Could you check a few things on this model? Use its own coordinates, in mm. Face numbers are marked on the shaded views. A direction names the side the tool comes from. Round coordinates to 2 decimals unless told otherwise and drop trailing zeros. Write each loop counter-clockwise with the first axis right and the second up, starting at its lowest first coordinate (ties: lowest second). Pieces come first, ordered by that corner, then holes. Notation, with made-up numbers: (-2.5, -23.5) -> (3.5, -23.5) arc R20 ccw to (3.5, 7.5) -> close; hole circle Ø4 at (39, 33). An arc over 180 degrees is marked (long way). Answer in a Markdown table with one row per item.
from build123d import *

# Parameters (mm, degrees)
BOSS_EXTRUDE7_DEPTH     = 6.5
BOSS_EXTRUDE8_START     = 1.7
BOSS_EXTRUDE8_DEPTH     = 1.7
CUT_EXTRUDE1_DEPTH      = 8.5
SKETCH6_W               = 12
SKETCH6_H               = 7.5
CUT_EXTRUDE2_DEPTH      = 8.5
CHAMFER1_SIZE           = 0.8
CHAMFER1_SIZE2          = 1.231891971
SKETCH7_R               = 0.4
CUT_EXTRUDE3_DEPTH      = 2
CUT_EXTRUDE3_DEPTH_BACK = 36.03740858
CHAMFER2_SIZE           = 0.5
CUT_EXTRUDE4_REACH      = 34.411
SKETCH12_R              = 0.8
BOSS_EXTRUDE9_DEPTH     = 0.5
CHAMFER3_SIZE           = 0.5


# Some blends are built 0.0001 mm under size
with BuildPart() as part:
    # Sketch1 → Boss-Extrude7 (new body)
    with BuildSketch(Plane(origin=(0, 0, 0), x_dir=(1, 0, 0), z_dir=(0, 1, 0))):
        with BuildLine():
            Line((0.8, 26.4), (19.9, 26.4))
            ThreePointArc((19.9, 26.4), (21.455634919, 25.755634919), (22.1, 24.2))
            Line((22.1, 24.2), (22.1, 0.8))
            ThreePointArc((22.1, 0.8), (21.455634919, -0.755634919), (19.9, -1.4))
            Line((19.9, -1.4), (0.8, -1.4))
            ThreePointArc((0.8, -1.4), (-0.755634919, -0.755634919), (-1.4, 0.8))
            Line((-1.4, 0.8), (-1.4, 24.2))
            ThreePointArc((-1.4, 24.2), (-0.755634919, 25.755634919), (0.8, 26.4))
        make_face()
        with BuildLine():
            Line((0.8, 25.2), (19.9, 25.2))
            ThreePointArc((19.9, 25.2), (20.607106781, 24.907106781), (20.9, 24.2))
            Line((20.9, 24.2), (20.9, 0.8))
            ThreePointArc((20.9, 0.8), (20.607106781, 0.092893219), (19.9, -0.2))
            Line((19.9, -0.2), (0.8, -0.2))
            ThreePointArc((0.8, -0.2), (0.092893219, 0.092893219), (-0.2, 0.8))
            Line((-0.2, 0.8), (-0.2, 24.2))
            ThreePointArc((-0.2, 24.2), (0.092893219, 24.907106781), (0.8, 25.2))
        make_face(mode=Mode.SUBTRACT)
    extrude(amount=BOSS_EXTRUDE7_DEPTH)

    # Sketch4 → Boss-Extrude8 (add)
    with BuildSketch(Plane.XZ.offset(BOSS_EXTRUDE8_START)):
        with BuildLine():
            Line((0.8, -26.4), (19.9, -26.4))
            ThreePointArc((19.9, -26.4), (21.455634919, -25.755634919), (22.1, -24.2))
            Line((22.1, -24.2), (22.1, -0.8))
            ThreePointArc((22.1, -0.8), (21.455634919, 0.755634919), (19.9, 1.4))
            Line((19.9, 1.4), (0.8, 1.4))
            ThreePointArc((0.8, 1.4), (-0.755634919, 0.755634919), (-1.4, -0.8))
            Line((-1.4, -0.8), (-1.4, -24.2))
            ThreePointArc((-1.4, -24.2), (-0.755634919, -25.755634919), (0.8, -26.4))
        make_face()
    extrude(amount=-BOSS_EXTRUDE8_DEPTH)

    # Sketch5 → Cut-Extrude1 (cut)
    with BuildSketch(Plane(origin=(0, 0, -26.4), x_dir=(-1, 0, 0), z_dir=(0, 0, -1))):
        with BuildLine():
            Line((-13.25, 2.9), (-7.45, 2.9))
            ThreePointArc((-7.45, 2.9), (-5.75, 1.2), (-7.45, -0.5))
            Line((-7.45, -0.5), (-13.25, -0.5))
            ThreePointArc((-13.25, -0.5), (-14.95, 1.2), (-13.25, 2.9))
        make_face()
    extrude(amount=-CUT_EXTRUDE1_DEPTH, mode=Mode.SUBTRACT)

    # Sketch6 → Cut-Extrude2 (cut)
    with BuildSketch(Plane(origin=(0, 0, 0), x_dir=(1, 0, 0), z_dir=(0, 1, 0))):
        with Locations((10.35, 9.85)):
            Rectangle(SKETCH6_W, SKETCH6_H)
    extrude(amount=-CUT_EXTRUDE2_DEPTH, mode=Mode.SUBTRACT)

    # Chamfer1
    chamfer1_edges = [part.edges().sort_by_distance(p)[0] for p in [
        (10.35, -1.7, -6.1),
        (16.35, -1.7, -9.85),
        (10.35, -1.7, -13.6),
        (4.35, -1.7, -9.85),
    ]]
    chamfer1_side = [part.faces().sort_by_distance(p)[0] for p in [
        (-0.498235424, -1.7, -25.498235424),
    ]]
    chamfer(chamfer1_edges, length=CHAMFER1_SIZE, length2=CHAMFER1_SIZE2, reference=chamfer1_side[0])

    # Cut-Sweep1: sweep along a path in Sketch9
    with BuildLine(Plane(origin=(0, 6.5, 0), x_dir=(1, 0, 0), z_dir=(0, 1, 0))) as cut_sweep1_path:
        Line((-1.4, 24.2), (-1.4, 0.8))
        ThreePointArc((-1.4, 0.8), (-0.755634919, -0.755634919), (0.8, -1.4))
        Line((0.8, -1.4), (19.9, -1.4))
        ThreePointArc((19.9, -1.4), (21.455634919, -0.755634919), (22.1, 0.8))
        Line((22.1, 0.8), (22.1, 24.2))
        ThreePointArc((22.1, 24.2), (21.455634919, 25.755634919), (19.9, 26.4))
        Line((19.9, 26.4), (0.8, 26.4))
        ThreePointArc((0.8, 26.4), (-0.755634919, 25.755634919), (-1.4, 24.2))
    # Sketch7 → Cut-Sweep1 (sweep, cut)
    with BuildSketch(Plane(origin=(0, 0, -16.4), x_dir=(-1, 0, 0), z_dir=(0, 0, -1))):
        with Locations((-20.9, 5.6)):
            Circle(SKETCH7_R)
    sweep(path=cut_sweep1_path.line, mode=Mode.SUBTRACT)

    # Sketch10 → Cut-Extrude3 (cut, two sides: drawn at the far end of the back side and taken through both)
    with BuildSketch(Plane(origin=(0, 0, 0), x_dir=(1, 0, 0), z_dir=(0, 1, 0)).offset(-CUT_EXTRUDE3_DEPTH_BACK)):
        with BuildLine():
            Line((15.905695732, 4), (13.405695732, 4))
            Line((13.405695732, 4), (13.405695732, 3.6))
            Line((13.405695732, 3.6), (15.905695732, 3.6))
            ThreePointArc((15.905695732, 3.6), (17.705695732, 1.8), (15.905695732, 0))
            Line((15.905695732, 0), (13.405695732, 0))
            Line((13.405695732, 0), (13.405695732, -0.4))
            Line((13.405695732, -0.4), (15.905695732, -0.4))
            ThreePointArc((15.905695732, -0.4), (18.105695732, 1.8), (15.905695732, 4))
        make_face()
    extrude(amount=CUT_EXTRUDE3_DEPTH + CUT_EXTRUDE3_DEPTH_BACK, mode=Mode.SUBTRACT)

    # Chamfer2
    # the kernel refuses this chamfer: 0.5 mm, written as the material it adds along each edge
    with BuildSketch(Plane(origin=(15.905695732, 2, -1.8), x_dir=(0, 0, 1), z_dir=(-1, 0, 0))) as chamfer2_piece_1_section:
        Polygon((2.2, -CHAMFER2_SIZE), (2.2 - CHAMFER2_SIZE, 0), (2.2, 0), align=None)
    chamfer2_piece_1 = revolve(axis=Axis((15.905695732, 2, -1.8), (0, 1, 0)), revolution_arc=58.108843161, mode=Mode.PRIVATE)
    chamfer2_piece_1 = split(chamfer2_piece_1, bisect_by=Plane(origin=(16.26277058, 1.786381102, 0.2), z_dir=(0, 0, 1)), keep=Keep.TOP, mode=Mode.PRIVATE)
    add(chamfer2_piece_1)
    with BuildSketch(Plane(origin=(12.119854238, 2, 0.4), x_dir=(0, -0.9996219169112968, 0.02749587661058638), z_dir=(1, 0, 0))) as chamfer2_piece_2_section:
        Polygon((CHAMFER2_SIZE * 0.999621916911, CHAMFER2_SIZE * 0.0274958766106), (-CHAMFER2_SIZE * 0.0274958766106, CHAMFER2_SIZE * 0.999621916911), (0, 0), align=None)
    chamfer2_piece_2 = extrude(amount=3.785841494, mode=Mode.PRIVATE)
    chamfer2_piece_2 = split(chamfer2_piece_2, bisect_by=Plane(origin=(14.374950242, 1.792648103, 0.2), z_dir=(0, 0, 1)), keep=Keep.TOP, mode=Mode.PRIVATE)
    add(chamfer2_piece_2)

    # Sketch11 → Cut-Extrude4 (cut, up to next)
    with BuildSketch(Plane(origin=(0, 0, -3.6), x_dir=(-1, 0, 0), z_dir=(0, 0, -1)), mode=Mode.PRIVATE) as cut_extrude4_sk1:
        Polygon((-13.405695732, 0), (-13.405695732, -1.1), (-14.505695732, 0), align=None)
    cut_extrude4_tool1 = extrude(cut_extrude4_sk1.sketch, amount=-CUT_EXTRUDE4_REACH, mode=Mode.PRIVATE) & part.part
    add(cut_extrude4_tool1.solids().sort_by_distance((13.772362, -0.366667, -3.6))[0], mode=Mode.SUBTRACT)

    # Sketch12 → Boss-Extrude9 (add)
    with BuildSketch(Plane(origin=(0, 0, 0), x_dir=(1, 0, 0), z_dir=(0, 1, 0))):
        with Locations(Location((15.905695732, 1.8, 0), (0, 0, 270))):
            Circle(SKETCH12_R)
    extrude(amount=BOSS_EXTRUDE9_DEPTH)

    # Chamfer3
    chamfer3_edges = [part.edges().sort_by_distance(p)[0] for p in [
        (15.905695732, 0, -2.6),
    ]]
    chamfer(chamfer3_edges, length=CHAMFER3_SIZE - 0.0001)  # a hair under: the kernel refuses the full size


solid = part.part
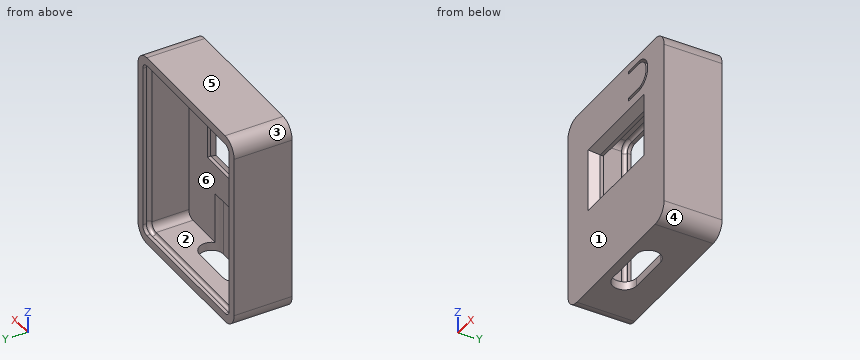
1) For the marked faces 5 and 6, which set-ups out of +Z, -Z, +X, -X, +Y, -Y let a thin tool reach every point of the face, with its end or its side?
Findings:
| item | result |
|---|---|
| face 5 | +Z, +X, -X, +Y, -Y |
| face 6 | +Y |
2) Imagine slicing it at C-C, the plane z = -19.75. Please give me the cut outline in (x, y).
Findings:
| item | result |
|---|---|
| outline | (-1.4, -1.7) -> (22.1, -1.7) -> (22.1, 6.5) -> (20.9, 6.5) -> (20.9, 6) arc R0.4 cw to (20.9, 5.2) -> (20.9, 0) -> (14.45, 0) arc R1.7 cw to (13.25, -0.5) -> (7.45, -0.5) arc R1.7 cw to (6.25, 0) -> (-0.2, 0) -> (-0.2, 5.2) arc R0.4 cw to (-0.2, 6) -> (-0.2, 6.5) -> (-1.4, 6.5) -> close |
3) Imagine slicing it at A-A, the plane y = 3.75. Please give me the cut outline in (x, z), plus the area to 3 significant figures.
Findings:
| item | result |
|---|---|
| outline | (-1.4, -24.2) arc R2.2 ccw to (0.8, -26.4) -> (19.9, -26.4) arc R2.2 ccw to (22.1, -24.2) -> (22.1, -0.8) arc R2.2 ccw to (19.9, 1.4) -> (0.8, 1.4) arc R2.2 ccw to (-1.4, -0.8) -> close; hole (-0.2, -24.2) arc R1 ccw to (0.8, -25.2) -> (19.9, -25.2) arc R1 ccw to (20.9, -24.2) -> (20.9, -0.8) arc R1 ccw to (19.9, 0.2) -> (0.8, 0.2) arc R1 ccw to (-0.2, -0.8) -> close |
| area | 114 mm^2 |
4) Imagine slicing it at B-B, the plane x = 8.5. Please give me the cut outline in (y, z).
Findings:
| item | result |
|---|---|
| outline | (-1.7, -26.4) -> (-0.5, -26.4) -> (-0.5, -17.9) -> (0, -17.9) -> (0, -13.6) -> (-0.47, -13.6) -> (-1.7, -14.4) -> close; (-1.7, -5.3) -> (-0.47, -6.1) -> (0, -6.1) -> (0, 0.2) -> (5.2, 0.2) arc R0.4 cw to (6, 0.2) -> (6.5, 0.2) -> (6.5, 1.4) -> (-1.7, 1.4) -> close; (2.9, -26.4) -> (6.5, -26.4) -> (6.5, -25.2) -> (6, -25.2) arc R0.4 cw to (5.2, -25.2) -> (2.9, -25.2) -> close |
5) Please list where these lines run through material, in increasing order: line 1 (Z direction, x = 19.25, y = 1.25); line 2 (X direction, y = 2, z = -4.5); line 3 (Y direction, x = 20.25, z = -15.5).
Findings:
| item | result |
|---|---|
| line 1 | z = -26.4 to -25.2, 0.2 to 1.4 |
| line 2 | x = -1.4 to -0.2, 20.9 to 22.1 |
| line 3 | y = -1.7 to 0 |
6) For pin 1 (1.7 mm diameter, centred on x = 11.5, z = -21, fed in from +Y); pin 2 (1.6 mm diameter, centred on x = 8.5, y = 1.5, fed in from -Z); pin 3 (0.8 mm diameter, centred on x = 16, z = -1.5, fed in from +Y), each with a flat end and sliding along its axis, tell me the tip position at first contact or that it passes through.
Findings:
| item | result |
|---|---|
| pin 1 | stops at y = -0.5 |
| pin 2 | stops at z = 0.2 |
| pin 3 | stops at y = 0.5 |
7) Imagine slicing it at D-D, the plane x = 18.5. Please give me the cut outline in (y, z).
Findings:
| item | result |
|---|---|
| outline | (-1.7, -26.4) -> (6.5, -26.4) -> (6.5, -25.2) -> (6, -25.2) arc R0.4 cw to (5.2, -25.2) -> (0, -25.2) -> (0, 0.2) -> (5.2, 0.2) arc R0.4 cw to (6, 0.2) -> (6.5, 0.2) -> (6.5, 1.4) -> (-1.7, 1.4) -> close |
8) Thinking about a two-plate mould opening in X: for the marked faces 1, 2, 3 and 4, which applies, +X half, -X half, draft (parallel to the pull), parting line (faces both ways), or undercut?
Findings:
| item | result |
|---|---|
| face 1 | draft |
| face 2 | undercut |
| face 3 | -X half |
| face 4 | +X half |
